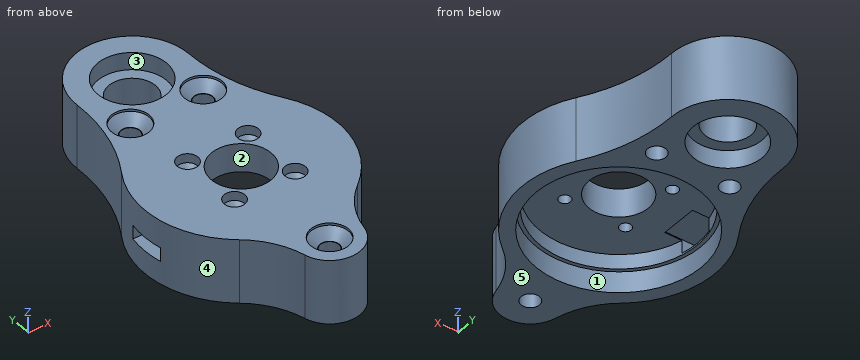
from build123d import *

# Parameters (mm, degrees)
CYLINDER015_R     = 2
CYLINDER015_DEPTH = 30
CYLINDER016_R     = 4.1
CYLINDER016_DEPTH = 0.5
CYLINDER017_R     = 2
CYLINDER017_DEPTH = 30
CYLINDER018_R     = 4.1
CYLINDER018_DEPTH = 0.5
CYLINDER013_R     = 2
CYLINDER013_DEPTH = 30
CYLINDER014_R     = 4.1
CYLINDER014_DEPTH = 0.5
CYLINDER001_R     = 2.4
CYLINDER001_DEPTH = 15.2
CYLINDER_R        = 17.2
CYLINDER_DEPTH    = 3.3
CYLINDER012_R     = 18
CYLINDER012_DEPTH = 11.1
BOX_W             = 10
BOX_H             = 8
BOX_DEPTH         = 3
CYLINDER007_R     = 7.5
CYLINDER007_DEPTH = 3.9
CYLINDER010_R     = 5.06
CYLINDER010_DEPTH = 15
CYLINDER004_R     = 7.5
CYLINDER004_DEPTH = 3.9
CYLINDER021_R     = 1.25
CYLINDER021_DEPTH = 8
CYLINDER022_R     = 2.25
CYLINDER022_DEPTH = 2.5
CYLINDER023_R     = 1.25
CYLINDER023_DEPTH = 8
CYLINDER024_R     = 2.25
CYLINDER024_DEPTH = 2.5
CYLINDER025_R     = 1.25
CYLINDER025_DEPTH = 8
CYLINDER026_R     = 2.25
CYLINDER026_DEPTH = 2.5
CYLINDER019_R     = 1.25
CYLINDER019_DEPTH = 8
CYLINDER020_R     = 2.25
CYLINDER020_DEPTH = 2.5
SKETCH_R          = 6.5
SKETCH_R_2        = 2.5
SKETCH_R_3        = 2
PAD_DEPTH         = 14


with BuildPart() as cone001:
    # Cone001 → Cone001 (revolve)
    with BuildSketch(Plane(origin=(0, -25.5, 18), x_dir=(1, 0, 0), z_dir=(0, -1, 0))):
        Polygon((0, 0), (2.1, 0), (4.1, 2), (0, 2), align=None)
    revolve(axis=Axis((0, -25.5, 18), (0, 0, 1)))


with BuildPart() as cylinders001:
    # Cylinder015 → Cylinder015 (new body)
    with BuildSketch(Plane(origin=(0, -25.5, -9.5), x_dir=(1, 0, 0), z_dir=(0, 0, 1))):
        Circle(CYLINDER015_R)
    extrude(amount=CYLINDER015_DEPTH)


with BuildPart() as fusion015:
    # Cylinder016 → Cylinder016 (new body)
    with BuildSketch(Plane(origin=(0, -25.5, 20), x_dir=(1, 0, 0), z_dir=(0, 0, 1))):
        Circle(CYLINDER016_R)
    extrude(amount=CYLINDER016_DEPTH)

    # Fusion015: union Cone001, CylinderS001
    add(cone001.part)
    add(cylinders001.part)


with BuildPart() as fusion015_1:
    # Fusion015 placement: moved
    add(fusion015.part.moved(Location((8, 47, 0.01))))


with BuildPart() as cone002:
    # Cone002 → Cone002 (revolve)
    with BuildSketch(Plane(origin=(0, -25.5, 18), x_dir=(1, 0, 0), z_dir=(0, -1, 0))):
        Polygon((0, 0), (2.1, 0), (4.1, 2), (0, 2), align=None)
    revolve(axis=Axis((0, -25.5, 18), (0, 0, 1)))


with BuildPart() as cylinders002:
    # Cylinder017 → Cylinder017 (new body)
    with BuildSketch(Plane(origin=(0, -25.5, -9.5), x_dir=(1, 0, 0), z_dir=(0, 0, 1))):
        Circle(CYLINDER017_R)
    extrude(amount=CYLINDER017_DEPTH)


with BuildPart() as fusion016:
    # Cylinder018 → Cylinder018 (new body)
    with BuildSketch(Plane(origin=(0, -25.5, 20), x_dir=(1, 0, 0), z_dir=(0, 0, 1))):
        Circle(CYLINDER018_R)
    extrude(amount=CYLINDER018_DEPTH)

    # Fusion016: union Cone002, CylinderS002
    add(cone002.part)
    add(cylinders002.part)


with BuildPart() as fusion016_1:
    # Fusion016 placement: moved
    add(fusion016.part.moved(Location((-8, 47, 0.01))))


with BuildPart() as cone:
    # Cone → Cone (revolve)
    with BuildSketch(Plane(origin=(0, -25.5, 18), x_dir=(1, 0, 0), z_dir=(0, -1, 0))):
        Polygon((0, 0), (2.1, 0), (4.1, 2), (0, 2), align=None)
    revolve(axis=Axis((0, -25.5, 18), (0, 0, 1)))


with BuildPart() as cylinders:
    # Cylinder013 → Cylinder013 (new body)
    with BuildSketch(Plane(origin=(0, -25.5, -9.5), x_dir=(1, 0, 0), z_dir=(0, 0, 1))):
        Circle(CYLINDER013_R)
    extrude(amount=CYLINDER013_DEPTH)


with BuildPart() as obj1:
    # Cylinder014 → Cylinder014 (new body)
    with BuildSketch(Plane(origin=(0, -25.5, 20), x_dir=(1, 0, 0), z_dir=(0, 0, 1))):
        Circle(CYLINDER014_R)
    extrude(amount=CYLINDER014_DEPTH)

    # Fusion014: union Cone, CylinderS
    add(cone.part)
    add(cylinders.part)


with BuildPart() as obj1_1:
    # Fusion014 placement: moved
    add(obj1.part.moved(Location((0, 0, 0.01))))

    # Fusion017: union Fusion015, Fusion016
    add(fusion015_1.part)
    add(fusion016_1.part)


with BuildPart() as motor_hole:
    # Cylinder001 → Cylinder001 (new body)
    with BuildSketch(Plane.XY):
        Circle(CYLINDER001_R)
    extrude(amount=CYLINDER001_DEPTH)


with BuildPart() as motor_stator:
    # Cylinder → Cylinder (new body)
    with BuildSketch(Plane.XY.offset(11)):
        Circle(CYLINDER_R)
    extrude(amount=CYLINDER_DEPTH)


with BuildPart() as motor:
    # Cylinder012 → Cylinder012 (new body)
    with BuildSketch(Plane.XY):
        Circle(CYLINDER012_R)
    extrude(amount=CYLINDER012_DEPTH)

    # Fusion011: union motor_stator
    add(motor_stator.part)

    # Cut: cut motor_hole
    add(motor_hole.part, mode=Mode.SUBTRACT)


with BuildPart() as wires:
    # Box → Box (new body)
    with BuildSketch(Plane(origin=(-23, -3.8, 11.5), x_dir=(1, 0, 0), z_dir=(0, 0, 1))):
        with Locations((5, 4)):
            Rectangle(BOX_W, BOX_H)
    extrude(amount=BOX_DEPTH)


with BuildPart() as bearing2:
    # Cylinder007 → Cylinder007 (new body)
    with BuildSketch(Plane.XY.offset(6.5)):
        Circle(CYLINDER007_R)
    extrude(amount=CYLINDER007_DEPTH)


with BuildPart() as bearingaxis:
    # Cylinder010 → Cylinder010 (new body)
    with BuildSketch(Plane.XY.offset(6)):
        Circle(CYLINDER010_R)
    extrude(amount=CYLINDER010_DEPTH)


with BuildPart() as bearings:
    # Cylinder004 → Cylinder004 (new body)
    with BuildSketch(Plane.XY.offset(16.7)):
        Circle(CYLINDER004_R)
    extrude(amount=CYLINDER004_DEPTH)

    # Fusion007: union Bearing2, BearingAxis
    add(bearing2.part)
    add(bearingaxis.part)


with BuildPart() as bearings_1:
    # Fusion007 placement: moved
    add(bearings.part.moved(Location((0, 31.5, 0))))


with BuildPart() as cylinder021:
    # Cylinder021 → Cylinder021 (new body)
    with BuildSketch(Plane.XY.offset(-10)):
        Circle(CYLINDER021_R)
    extrude(amount=CYLINDER021_DEPTH)


with BuildPart() as cylinder022:
    # Cylinder022 → Cylinder022 (new body)
    with BuildSketch(Plane.XY.offset(-2)):
        Circle(CYLINDER022_R)
    extrude(amount=CYLINDER022_DEPTH)


with BuildPart() as fusion020:
    # Cone004 → Cone004 (revolve)
    with BuildSketch(Plane(origin=(0, 0, -3), x_dir=(1, 0, 0), z_dir=(0, -1, 0))):
        Polygon((0, 0), (1.25, 0), (2.25, 1), (0, 1), align=None)
    revolve(axis=Axis((0, 0, -3), (0, 0, 1)))

    # Fusion020: union Cylinder021, Cylinder022
    add(cylinder021.part)
    add(cylinder022.part)


with BuildPart() as fusion020_1:
    # Fusion020 placement: moved
    add(fusion020.part.moved(Location((6.65, 6.785, 20.51))))


with BuildPart() as cylinder023:
    # Cylinder023 → Cylinder023 (new body)
    with BuildSketch(Plane.XY.offset(-10)):
        Circle(CYLINDER023_R)
    extrude(amount=CYLINDER023_DEPTH)


with BuildPart() as cylinder024:
    # Cylinder024 → Cylinder024 (new body)
    with BuildSketch(Plane.XY.offset(-2)):
        Circle(CYLINDER024_R)
    extrude(amount=CYLINDER024_DEPTH)


with BuildPart() as fusion021:
    # Cone005 → Cone005 (revolve)
    with BuildSketch(Plane(origin=(0, 0, -3), x_dir=(1, 0, 0), z_dir=(0, -1, 0))):
        Polygon((0, 0), (1.25, 0), (2.25, 1), (0, 1), align=None)
    revolve(axis=Axis((0, 0, -3), (0, 0, 1)))

    # Fusion021: union Cylinder023, Cylinder024
    add(cylinder023.part)
    add(cylinder024.part)


with BuildPart() as fusion021_1:
    # Fusion021 placement: moved
    add(fusion021.part.moved(Location((-6.65, -6.79, 20.51))))


with BuildPart() as cylinder025:
    # Cylinder025 → Cylinder025 (new body)
    with BuildSketch(Plane.XY.offset(-10)):
        Circle(CYLINDER025_R)
    extrude(amount=CYLINDER025_DEPTH)


with BuildPart() as cylinder026:
    # Cylinder026 → Cylinder026 (new body)
    with BuildSketch(Plane.XY.offset(-2)):
        Circle(CYLINDER026_R)
    extrude(amount=CYLINDER026_DEPTH)


with BuildPart() as fusion022:
    # Cone006 → Cone006 (revolve)
    with BuildSketch(Plane(origin=(0, 0, -3), x_dir=(1, 0, 0), z_dir=(0, -1, 0))):
        Polygon((0, 0), (1.25, 0), (2.25, 1), (0, 1), align=None)
    revolve(axis=Axis((0, 0, -3), (0, 0, 1)))

    # Fusion022: union Cylinder025, Cylinder026
    add(cylinder025.part)
    add(cylinder026.part)


with BuildPart() as fusion022_1:
    # Fusion022 placement: moved
    add(fusion022.part.moved(Location((6.65, -6.79, 20.51))))


with BuildPart() as cylinder019:
    # Cylinder019 → Cylinder019 (new body)
    with BuildSketch(Plane.XY.offset(-10)):
        Circle(CYLINDER019_R)
    extrude(amount=CYLINDER019_DEPTH)


with BuildPart() as cylinder020:
    # Cylinder020 → Cylinder020 (new body)
    with BuildSketch(Plane.XY.offset(-2)):
        Circle(CYLINDER020_R)
    extrude(amount=CYLINDER020_DEPTH)


with BuildPart() as obj2:
    # Cone003 → Cone003 (revolve)
    with BuildSketch(Plane(origin=(0, 0, -3), x_dir=(1, 0, 0), z_dir=(0, -1, 0))):
        Polygon((0, 0), (1.25, 0), (2.25, 1), (0, 1), align=None)
    revolve(axis=Axis((0, 0, -3), (0, 0, 1)))

    # Fusion019: union Cylinder019, Cylinder020
    add(cylinder019.part)
    add(cylinder020.part)


with BuildPart() as obj2_1:
    # Fusion019 placement: moved
    add(obj2.part.moved(Location((-6.65, 6.785, 20.51))))

    # Fusion023: union Fusion020, Fusion021, Fusion022
    add(fusion020_1.part)
    add(fusion021_1.part)
    add(fusion022_1.part)

    # Fusion024: union obj1, Motor, Wires, Bearings
    add(obj1_1.part)
    add(motor.part)
    add(wires.part)
    add(bearings_1.part)


with BuildPart() as hip:
    # Sketch → Pad (new body)
    with BuildSketch(Plane.XY.offset(14)):
        with BuildLine():
            ThreePointArc((12.20842, 31.303575), (0, 43.71), (-12.20842, 31.303575))
            ThreePointArc((-17.815108, 11.11854), (-13.553348, 20.805961), (-12.20842, 31.303575))
            ThreePointArc((-17.815108, 11.11854), (-20.685819, -3.61896), (-12.982142, -16.506483))
            ThreePointArc((-6.502297, -26.893782), (-8.833051, -21.132971), (-12.982142, -16.506483))
            ThreePointArc((-6.502297, -26.893782), (0, -32.15), (6.502297, -26.893782))
            ThreePointArc((12.982142, -16.506483), (8.833051, -21.132971), (6.502297, -26.893782))
            ThreePointArc((12.982142, -16.506483), (20.685819, -3.61896), (17.815108, 11.11854))
            ThreePointArc((12.20842, 31.303575), (13.553348, 20.805961), (17.815108, 11.11854))
        make_face()
        Circle(SKETCH_R, mode=Mode.SUBTRACT)
        with Locations((0, 31.5)):
            Circle(SKETCH_R_2, mode=Mode.SUBTRACT)
        with Locations((0, -25.5)):
            Circle(SKETCH_R_3, mode=Mode.SUBTRACT)
    extrude(amount=PAD_DEPTH)


with BuildPart() as hip_1:
    # Body placement: moved
    add(hip.part.moved(Location((0, 0, -7.5))))

    # Cut004: cut obj2
    add(obj2_1.part, mode=Mode.SUBTRACT)


solid = hip_1.part
CAD build for the part. Positions are in the model's coordinates, mm. Face numbers are marked on the shaded views. A direction names the side the tool comes from. Give positions to 0.01 mm unless a question says otherwise; leave off trailing zeros. Order: outer loops, then holes, each group sorted by start corner. A loop starts at its lowest first (then second) coordinate and runs counter-clockwise, first axis right, second up. Notation, with made-up numbers: (49.25, 65) - (70.25, 65) arc R31 ccw to (70.25, 103) - close; hole circle Ø6 at (68.25, -19.5). An arc over 180 degrees is marked (long way). Write each question's results on one line, items separated by ' | '.
1. Probe L1, parallel to Y at x = 4.5, z = 15.25; L2, parallel to X at y = 31.5, z = 12.5; L3, parallel to Y at x = 5, z = 18.5. List the from-to ranges inside material, lowest first. Write a range as from..to.
Calculated:
L1: y = -30.4..-4.69, 4.69..29.19, 33.81..42.85 | L2: x = -12.21..-5.06, 5.06..12.21 | L3: y = -29.88..-8.3, -5.28..-4.15, 4.15..5.27, 8.3..25.91, 37.09..42.64
2. Pin check, flat tips, straight feed: pin 1 (2.5 mm diameter, centred on x = -17.5, z = 13, fed in from -Y); pin 2 (2.5 mm diameter, centred on x = -16.5, y = 0.5, fed in from -Z); pin 3 (9 mm diameter, centred on x = 0, y = 31.5, fed in from -Z); pin 4 (8 mm diameter, centred on x = 7, z = 18.5, fed in from +Y). Stop position of each tip, or through.
Calculated:
pin 1: stops at y = -13.3 | pin 2: stops at z = 11.1 | pin 3: passes through | pin 4: stops at y = 43.34
3. Pull direction X, two halves, no side cores. Call the marked faces 3, 4 and 5: released by +X, released by -X, zero draft, split by the parting line, or undercut.
Calculated:
face 3: undercut | face 4: released by -X | face 5: zero draft
4. Saw through at C-C on z = 12.5. List the corners of the cut face in (x, y), and give its area (3 significant figures).
Calculated:
outline: (-20.65, -3.8) arc R21 ccw to (-12.98, -16.51) arc R18.02 cw to (-6.5, -26.89) arc R6.65 ccw to (6.5, -26.89) arc R18.02 cw to (12.98, -16.51) arc R21 ccw to (17.82, 11.12) arc R37 cw to (12.21, 31.3) arc R12.21 ccw (long way) to (-12.21, 31.3) arc R37 cw to (-17.82, 11.12) arc R21 ccw to (-20.58, 4.2) - (-16.68, 4.2) arc R17.2 cw (long way) to (-16.77, -3.8) - close; hole circle Ø4 at (-8, 21.5); hole circle Ø10.12 at (0, 31.5); hole circle Ø4 at (0, -25.5); hole circle Ø4 at (8, 21.5) | area: 1,020 mm2
5. 3-axis set-ups, long thin cutter, end or side, ignore diameter. For the marked faces 1 and 2: which of +Z, -Z, +X, -X, +Y, -Y reach the whole face in a straight line?
Calculated:
face 1: -Z | face 2: +Z, -Z
6. Saw through at B-B on y = -25.5. List the corners of the cut face in (x, z), and give its area (3 significant figures).
Calculated:
outline: (-6.86, 6.5) - (-2, 6.5) - (-2, 18.01) - (-2.1, 18.01) - (-4.1, 20.01) - (-4.1, 20.5) - (-6.86, 20.5) - close; (2, 6.5) - (6.86, 6.5) - (6.86, 20.5) - (4.1, 20.5) - (4.1, 20.01) - (2.1, 18.01) - (2, 18.01) - close | area: 130 mm2
7. Saw through at A-A on y = 0. List the corners of the cut face in (x, z).
Calculated:
outline: (-21, 6.5) - (-18, 6.5) - (-18, 11.1) - (-17.2, 11.1) - (-17.2, 11.5) - (-21, 11.5) - close; (-21, 14.5) - (-13, 14.5) - (-13, 14.3) - (-6.5, 14.3) - (-6.5, 20.5) - (-21, 20.5) - close; (6.5, 14.3) - (17.2, 14.3) - (17.2, 11.1) - (18, 11.1) - (18, 6.5) - (21, 6.5) - (21, 20.5) - (6.5, 20.5) - close
8. Saw through at D-D on x = 15. List the corners of the cut face in (y, z), and give its area (3 significant figures).
Calculated:
outline: (-14.7, 6.5) - (-9.95, 6.5) - (-9.95, 11.1) - (-8.42, 11.1) - (-8.42, 14.3) - (8.42, 14.3) - (8.42, 11.1) - (9.95, 11.1) - (9.95, 6.5) - (16.6, 6.5) - (16.6, 20.5) - (-14.7, 20.5) - close | area: 293 mm2
